```python
from build123d import *

# Parameters (mm, degrees)
F2_W      = 20
F2_H      = 16
F2_R      = 1.4
F3_DEPTH  = 11.5
F4_SIZE   = 0.5
F7_R      = 2.5
F8_DEPTH  = 3.5
F9_ANGLE  = -90
F10_R     = 4
F11_DEPTH = 10


with BuildPart() as f1:
    # F0 (on Front) → F1 (revolve)
    with BuildSketch(Plane.XZ):
        Polygon((8, 42.7), (0, 42.7), (0, 0), (0, -2.1), (1.4, -2.1), (1.4, 0), (11.1, 0), (11.1, 1), (7.187217, 1), (7.055984, 2.5), (11.1, 2.5), (11.1, 3.5), (6.968495, 3.5), (6.837262, 5), (11.1, 5), (11.1, 6), (6.749773, 6), (6.61854, 7.5), (11.1, 7.5), (11.1, 8.5), (6.531052, 8.5), (6.399819, 10), (11.1, 10), (11.1, 11), (6.31233, 11), (6.181097, 12.5), (11.1, 12.5), (11.1, 13.5), (6.093608, 13.5), (5.962375, 15), (11.1, 15), (11.1, 16), (5.874887, 16), (5.743654, 17.5), (11.1, 17.5), (11.1, 18.5), (5.656165, 18.5), (5.524932, 20), (11.1, 20), (11.1, 21), (5.437443, 21), (5.30621, 22.5), (11.1, 22.5), (11.1, 23.5), (5.218722, 23.5), (5.087489, 25), (11.1, 25), (11.1, 26), (3.490466, 26), (3.490466, 27.5), (8, 27.5), (8, 28.5), (3.490466, 28.5), (3.490466, 30), (8, 30), (8, 33), (6, 33), (6, 39), (8, 39), align=None)
    revolve(axis=Axis((0, 0, 21.35), (0, 0, 1)))

    # F2 (on face) → F3 (join)
    with BuildSketch(Plane(origin=(0, 0, -2.1), x_dir=(1, 0, 0), z_dir=(0, 0, -1))):
        with Locations((-5.5, 0)):
            Rectangle(F2_W, F2_H)
        Circle(F2_R, mode=Mode.SUBTRACT)
        Circle(F2_R)
    extrude(amount=F3_DEPTH)

    # F4
    f4_edges = [f1.edges().sort_by_distance(p)[0] for p in [
        (4.5, -8, -7.85),
        (-15.5, -8, -7.85),
        (-5.5, -8, -2.1),
        (-5.5, -8, -13.6),
        (4.5, 8, -7.85),
        (4.5, 0, -2.1),
        (4.5, 0, -13.6),
        (-15.5, 8, -7.85),
        (-5.5, 8, -2.1),
        (-5.5, 8, -13.6),
        (-15.5, 0, -2.1),
        (-15.5, 0, -13.6),
    ]]
    chamfer(f4_edges, length=F4_SIZE)

    # F5 (on Front) → F6 (revolve)
    with BuildSketch(Plane.XZ):
        Polygon((2.5, -7.1), (0, -7.1), (0, -19.6), (0.5, -19.6), (1.900415, -17.6), (2.5, -17.6), (2.5, -14.6), align=None)
    revolve(axis=Axis((0, 0, -13.35), (0, 0, -1)))

    # F7 (on face) → F8 (join)
    with BuildSketch(Plane(origin=(0, 0, -17.6), x_dir=(1, 0, 0), z_dir=(0, 0, -1))):
        Polygon((2.020726, -3.5), (4.041452, 0), (2.020726, 3.5), (-2.020726, 3.5), (-4.041452, 0), (-2.020726, -3.5), align=None)
        Circle(F7_R, mode=Mode.SUBTRACT)
    extrude(amount=-F8_DEPTH)


with BuildPart() as f1_1:
    # F9: moved
    add(f1.part.rotate(Axis((0, 0, 21.35), (0, 0, 1)), F9_ANGLE))

    # F10 (on face) → F11 (cut)
    with BuildSketch(Plane.XY.offset(42.7)):
        Circle(F10_R)
    extrude(amount=-F11_DEPTH, mode=Mode.SUBTRACT)


solid = f1_1.part
```
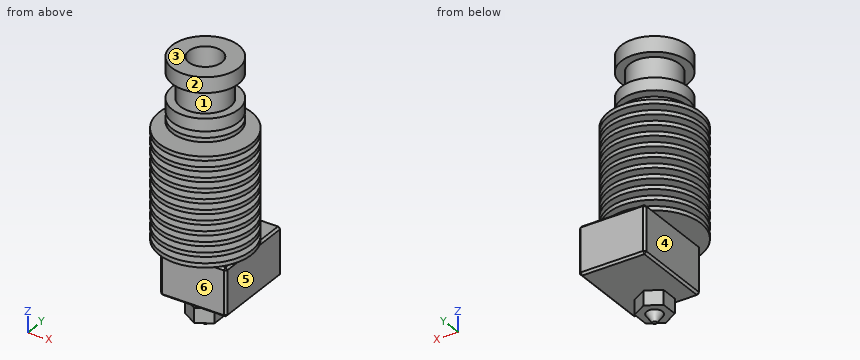
Verification items for the finished model (mm, model axes). Face numbers are marked on the shaded views. A direction names the side the tool comes from. Give positions to 0.01 mm unless a question says otherwise; leave off trailing zeros.
1. Mould release check, pull along Z, two halves, no side actions. Record for the marked faces 1, 2 and 3: released by +Z, released by -Z, zero draft, split by the parting line, or undercut.
2. Section check A-A, the plane y = 9.5. Count the separate pieces of the cut face and the enclosed holes in it, then the cut area to 3 significant figures.
3. Set-up check for the marked faces 4, 5 and 6: record each of +Z, -Z, +X, -X, +Y, -Y from which the full face is reachable in a straight line by a thin tool's end or side.
4. Thickness scan on line 1 (Z direction, x = 1.5, y = 3.75); line 2 (X direction, y = 5.75, z = -9); line 3 (Z direction, x = 1, y = 14.25). Record the ranges inside material, lowest first.
5. Go/stop test with flat-tipped pins: pin 1 Ø10 at (x, z) = (1.5, -9.5) entering from -Y; pin 2 Ø12 at (x, z) = (5, 30.5) entering from -Y; pin 3 Ø6.5 at (x, y) = (-4, 0) entering from -Z. Record where each tip stops, or that it passes through.
Geometry says:
1. face 1: undercut
1. face 2: zero draft
1. face 3: released by +Z
2. separate pieces: 12
2. enclosed holes: 0
2. area: 310 mm2
3. face 4: -Z, -X, +Y, -Y
3. face 5: -Z, +X, +Y, -Y
3. face 6: -Z, +X, -X, -Y
4. line 1: z = -13.6 to -2.1, 0 to 26, 27.5 to 28.5, 30 to 42.7
4. line 2: x = -8 to 8
4. line 3: z = -13.6 to -2.1
5. pin 1: stops at y = -4.5
5. pin 2: stops at y = -11.05
5. pin 3: stops at z = -19.24
